```python
from build123d import *

# Parameters (mm, degrees)
SKETCH_1_W          = 100
SKETCH_1_H          = 100
SKETCH_1_R          = 6.5
EXTRUDE_1_DEPTH     = 4.4
FILLET_1_R          = 10
CUT_EXTRUDE_1_REACH = 6.4
SKETCH_2_R          = 1.6
SKETCH_2_W          = 15
SKETCH_2_H          = 4.4
SKETCH_2_W_2        = 4.4
SKETCH_2_H_2        = 15


with BuildPart() as part:
    # 草图1 → 凸台-拉伸1 (new body)
    with BuildSketch(Plane(origin=(0, 0, 0), x_dir=(1, 0, 0), z_dir=(0, 1, 0))):
        Rectangle(SKETCH_1_W, SKETCH_1_H)
        Circle(SKETCH_1_R, mode=Mode.SUBTRACT)
    extrude(amount=EXTRUDE_1_DEPTH)

    # 圆角1
    fillet_1_edges = [part.edges().sort_by_distance(p)[0] for p in [
        (50, 2.2, 50),
        (-50, 2.2, 50),
        (-50, 2.2, -50),
        (50, 2.2, -50),
    ]]
    fillet(fillet_1_edges, radius=FILLET_1_R)

    # 草图2 → 切除-拉伸1 (cut, up to next)
    with BuildSketch(Plane(origin=(0, 4.4, 0), x_dir=(1, 0, 0), z_dir=(0, 1, 0)), mode=Mode.PRIVATE) as cut_extrude_1_sk1:
        with Locations((40, 40)):
            Circle(SKETCH_2_R)
    cut_extrude_1_tool1 = extrude(cut_extrude_1_sk1.sketch, amount=-CUT_EXTRUDE_1_REACH, mode=Mode.PRIVATE) & part.part
    add(cut_extrude_1_tool1.solids().sort_by_distance((40, 4.4, -40))[0], mode=Mode.SUBTRACT)
    # 草图2 → 切除-拉伸1 (cut, up to next)
    with BuildSketch(Plane(origin=(0, 4.4, 0), x_dir=(1, 0, 0), z_dir=(0, 1, 0)), mode=Mode.PRIVATE) as cut_extrude_1_sk2:
        with Locations((40, -40)):
            Circle(SKETCH_2_R)
    cut_extrude_1_tool2 = extrude(cut_extrude_1_sk2.sketch, amount=-CUT_EXTRUDE_1_REACH, mode=Mode.PRIVATE) & part.part
    add(cut_extrude_1_tool2.solids().sort_by_distance((40, 4.4, 40))[0], mode=Mode.SUBTRACT)
    # 草图2 → 切除-拉伸1 (cut, up to next)
    with BuildSketch(Plane(origin=(0, 4.4, 0), x_dir=(1, 0, 0), z_dir=(0, 1, 0)), mode=Mode.PRIVATE) as cut_extrude_1_sk3:
        with Locations((-40, -40)):
            Circle(SKETCH_2_R)
    cut_extrude_1_tool3 = extrude(cut_extrude_1_sk3.sketch, amount=-CUT_EXTRUDE_1_REACH, mode=Mode.PRIVATE) & part.part
    add(cut_extrude_1_tool3.solids().sort_by_distance((-40, 4.4, 40))[0], mode=Mode.SUBTRACT)
    # 草图2 → 切除-拉伸1 (cut, up to next)
    with BuildSketch(Plane(origin=(0, 4.4, 0), x_dir=(1, 0, 0), z_dir=(0, 1, 0)), mode=Mode.PRIVATE) as cut_extrude_1_sk4:
        with Locations((-40, 40)):
            Circle(SKETCH_2_R)
    cut_extrude_1_tool4 = extrude(cut_extrude_1_sk4.sketch, amount=-CUT_EXTRUDE_1_REACH, mode=Mode.PRIVATE) & part.part
    add(cut_extrude_1_tool4.solids().sort_by_distance((-40, 4.4, -40))[0], mode=Mode.SUBTRACT)
    # 草图2 → 切除-拉伸1 (cut, up to next)
    with BuildSketch(Plane(origin=(0, 4.4, 0), x_dir=(1, 0, 0), z_dir=(0, 1, 0)), mode=Mode.PRIVATE) as cut_extrude_1_sk5:
        with Locations((-16.5, 41.8)):
            Rectangle(SKETCH_2_W, SKETCH_2_H)
    cut_extrude_1_tool5 = extrude(cut_extrude_1_sk5.sketch, amount=-CUT_EXTRUDE_1_REACH, mode=Mode.PRIVATE) & part.part
    add(cut_extrude_1_tool5.solids().sort_by_distance((-16.5, 4.4, -41.8))[0], mode=Mode.SUBTRACT)
    # 草图2 → 切除-拉伸1 (cut, up to next)
    with BuildSketch(Plane(origin=(0, 4.4, 0), x_dir=(1, 0, 0), z_dir=(0, 1, 0)), mode=Mode.PRIVATE) as cut_extrude_1_sk6:
        with Locations((16.5, 41.8)):
            Rectangle(SKETCH_2_W, SKETCH_2_H)
    cut_extrude_1_tool6 = extrude(cut_extrude_1_sk6.sketch, amount=-CUT_EXTRUDE_1_REACH, mode=Mode.PRIVATE) & part.part
    add(cut_extrude_1_tool6.solids().sort_by_distance((16.5, 4.4, -41.8))[0], mode=Mode.SUBTRACT)
    # 草图2 → 切除-拉伸1 (cut, up to next)
    with BuildSketch(Plane(origin=(0, 4.4, 0), x_dir=(1, 0, 0), z_dir=(0, 1, 0)), mode=Mode.PRIVATE) as cut_extrude_1_sk7:
        with Locations((41.8, -16.5)):
            Rectangle(SKETCH_2_W_2, SKETCH_2_H_2)
    cut_extrude_1_tool7 = extrude(cut_extrude_1_sk7.sketch, amount=-CUT_EXTRUDE_1_REACH, mode=Mode.PRIVATE) & part.part
    add(cut_extrude_1_tool7.solids().sort_by_distance((41.8, 4.4, 16.5))[0], mode=Mode.SUBTRACT)
    # 草图2 → 切除-拉伸1 (cut, up to next)
    with BuildSketch(Plane(origin=(0, 4.4, 0), x_dir=(1, 0, 0), z_dir=(0, 1, 0)), mode=Mode.PRIVATE) as cut_extrude_1_sk8:
        with Locations((41.8, 16.5)):
            Rectangle(SKETCH_2_W_2, SKETCH_2_H_2)
    cut_extrude_1_tool8 = extrude(cut_extrude_1_sk8.sketch, amount=-CUT_EXTRUDE_1_REACH, mode=Mode.PRIVATE) & part.part
    add(cut_extrude_1_tool8.solids().sort_by_distance((41.8, 4.4, -16.5))[0], mode=Mode.SUBTRACT)
    # 草图2 → 切除-拉伸1 (cut, up to next)
    with BuildSketch(Plane(origin=(0, 4.4, 0), x_dir=(1, 0, 0), z_dir=(0, 1, 0)), mode=Mode.PRIVATE) as cut_extrude_1_sk9:
        with Locations((-16.5, -41.8)):
            Rectangle(SKETCH_2_W, SKETCH_2_H)
    cut_extrude_1_tool9 = extrude(cut_extrude_1_sk9.sketch, amount=-CUT_EXTRUDE_1_REACH, mode=Mode.PRIVATE) & part.part
    add(cut_extrude_1_tool9.solids().sort_by_distance((-16.5, 4.4, 41.8))[0], mode=Mode.SUBTRACT)
    # 草图2 → 切除-拉伸1 (cut, up to next)
    with BuildSketch(Plane(origin=(0, 4.4, 0), x_dir=(1, 0, 0), z_dir=(0, 1, 0)), mode=Mode.PRIVATE) as cut_extrude_1_sk10:
        with Locations((16.5, -41.8)):
            Rectangle(SKETCH_2_W, SKETCH_2_H)
    cut_extrude_1_tool10 = extrude(cut_extrude_1_sk10.sketch, amount=-CUT_EXTRUDE_1_REACH, mode=Mode.PRIVATE) & part.part
    add(cut_extrude_1_tool10.solids().sort_by_distance((16.5, 4.4, 41.8))[0], mode=Mode.SUBTRACT)
    # 草图2 → 切除-拉伸1 (cut, up to next)
    with BuildSketch(Plane(origin=(0, 4.4, 0), x_dir=(1, 0, 0), z_dir=(0, 1, 0)), mode=Mode.PRIVATE) as cut_extrude_1_sk11:
        with Locations((-41.8, 16.5)):
            Rectangle(SKETCH_2_W_2, SKETCH_2_H_2)
    cut_extrude_1_tool11 = extrude(cut_extrude_1_sk11.sketch, amount=-CUT_EXTRUDE_1_REACH, mode=Mode.PRIVATE) & part.part
    add(cut_extrude_1_tool11.solids().sort_by_distance((-41.8, 4.4, -16.5))[0], mode=Mode.SUBTRACT)
    # 草图2 → 切除-拉伸1 (cut, up to next)
    with BuildSketch(Plane(origin=(0, 4.4, 0), x_dir=(1, 0, 0), z_dir=(0, 1, 0)), mode=Mode.PRIVATE) as cut_extrude_1_sk12:
        with Locations((-41.8, -16.5)):
            Rectangle(SKETCH_2_W_2, SKETCH_2_H_2)
    cut_extrude_1_tool12 = extrude(cut_extrude_1_sk12.sketch, amount=-CUT_EXTRUDE_1_REACH, mode=Mode.PRIVATE) & part.part
    add(cut_extrude_1_tool12.solids().sort_by_distance((-41.8, 4.4, 16.5))[0], mode=Mode.SUBTRACT)


solid = part.part
```
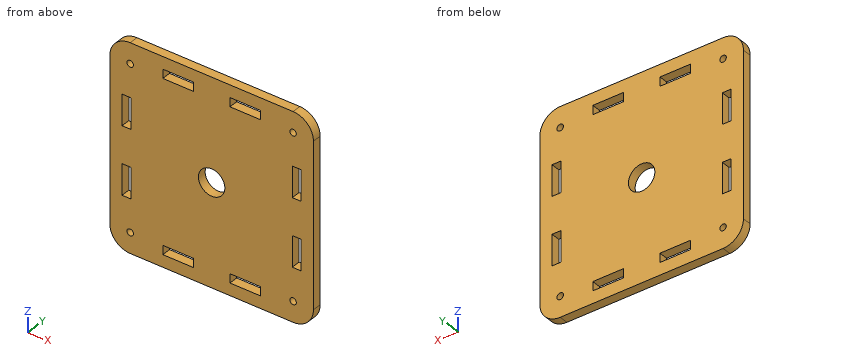
Part model, mm, in its own coordinate system. Coordinates: 2 decimals unless noted, no trailing zeros. Loops run counter-clockwise (first coordinate to the right, second up) from the corner with the lowest first, then second, coordinate; pieces in that order, holes last. Notation, with made-up numbers: (0, 11) - (18, 11) arc R16 ccw to (18, 37) - close; hole circle Ø5 at (-23.75, 5). An arc over 180 degrees is marked (long way). Write item = value, one per line. Start each with the question number.
Item 1: Cut at A-A, the plane x = 0. Give the cut face in (y, z), and give its area (3 significant figures).
Item 2: Cut at B-B, the plane z = -12. Give the cut face in (x, y).
Item 3: Cut at C-C, the plane x = 14. Give the cut face in (y, z), and give its area (3 significant figures).
Item 4: Flat gauge pins, fed straight in: pin 1 Ø2 at (x, y) = (-41, 3) entering from -Z; pin 2 Ø1.3 at (x, y) = (41.5, 2) entering from +Z. Where does each tip first touch, or does it go through?
Item 5: Cut at D-D, the plane y = 1.25. State how many separate pieces and enclosed holes the cut face has, and give its area (3 significant figures).
Item 6: Wall check: L1, parallel to X at y = 3.2, z = -18.5; L2, parallel to X at y = 3.1, z = -40. Give the ranges that are in metal, low to high. Write a range as from..to.
The answers:
q1.outline = (0, -50) - (4.4, -50) - (4.4, -6.5) - (0, -6.5) - close; (0, 6.5) - (4.4, 6.5) - (4.4, 50) - (0, 50) - close
q1.area = 383 mm2
q2.outline = (-50, 0) - (-44, 0) - (-44, 4.4) - (-50, 4.4) - close; (-39.6, 0) - (39.6, 0) - (39.6, 4.4) - (-39.6, 4.4) - close; (44, 0) - (50, 0) - (50, 4.4) - (44, 4.4) - close
q3.outline = (0, -50) - (4.4, -50) - (4.4, -44) - (0, -44) - close; (0, -39.6) - (4.4, -39.6) - (4.4, 39.6) - (0, 39.6) - close; (0, 44) - (4.4, 44) - (4.4, 50) - (0, 50) - close
q3.area = 401 mm2
q4.pin_1 = -50
q4.pin_2 = 49.96
q5.separate_pieces = 1
q5.enclosed_holes = 13
q5.area = 9,220 mm2
q6.L1 = -50..-44, -39.6..39.6, 44..50
q6.L2 = -50..-41.6, -38.4..-24, -9..9, 24..38.4, 41.6..50
